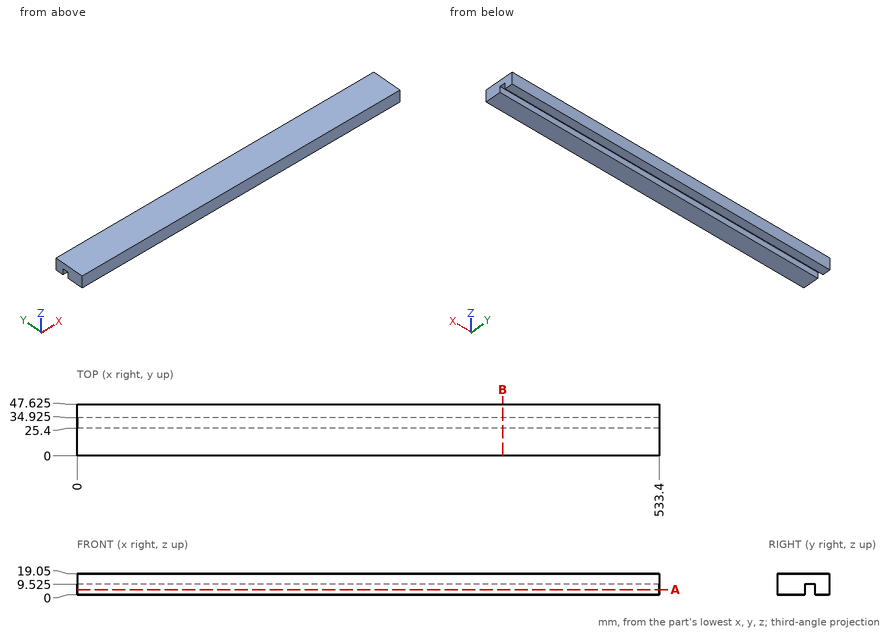
Job drawing, mm, ordinate dimensions from the low corner. One solid piece. Coordinates: 2 decimals unless noted, no trailing zeros. Order: outer loops, then holes, each group sorted by start corner. A loop starts at its lowest first (then second) coordinate and runs counter-clockwise, first axis right, second up. Notation, with made-up numbers: M 49.5,62 L 101.5,62 A15 ccw 101.5,67 Z; hole C 64.5,-40 d10. An arc over 180 degrees is marked long. One line per question, with ' | ' between items.
Q1. Slice it at A-A (z = 4.75). Give the cut face in (x, y) (3 decimals), and give its area (3 significant figures).
A:
outline: M 0,0 L 533.4,0 L 533.4,25.4 L 0,25.4 Z; M 0,34.925 L 533.4,34.925 L 533.4,47.625 L 0,47.625 Z | area: 20,300 mm^2
Q2. Slice it at B-B (x = 390). Give the cut face in (y, z) (3 decimals), and give its area (3 significant figures).
A:
outline: M 0,0 L 25.4,0 L 25.4,9.525 L 34.925,9.525 L 34.925,0 L 47.625,0 L 47.625,19.05 L 0,19.05 Z | area: 817 mm^2
Q3. Drill centre lines: line 1 (Y direction, x = 155.5, z = 6.75) (3 decimals); line 2 (Z direction, x = 208, y = 30) (3 decimals). Where is each one in solid material? Low to high.
A:
line 1: y = 0 to 25.4, 34.925 to 47.625 | line 2: z = 9.525 to 19.05
